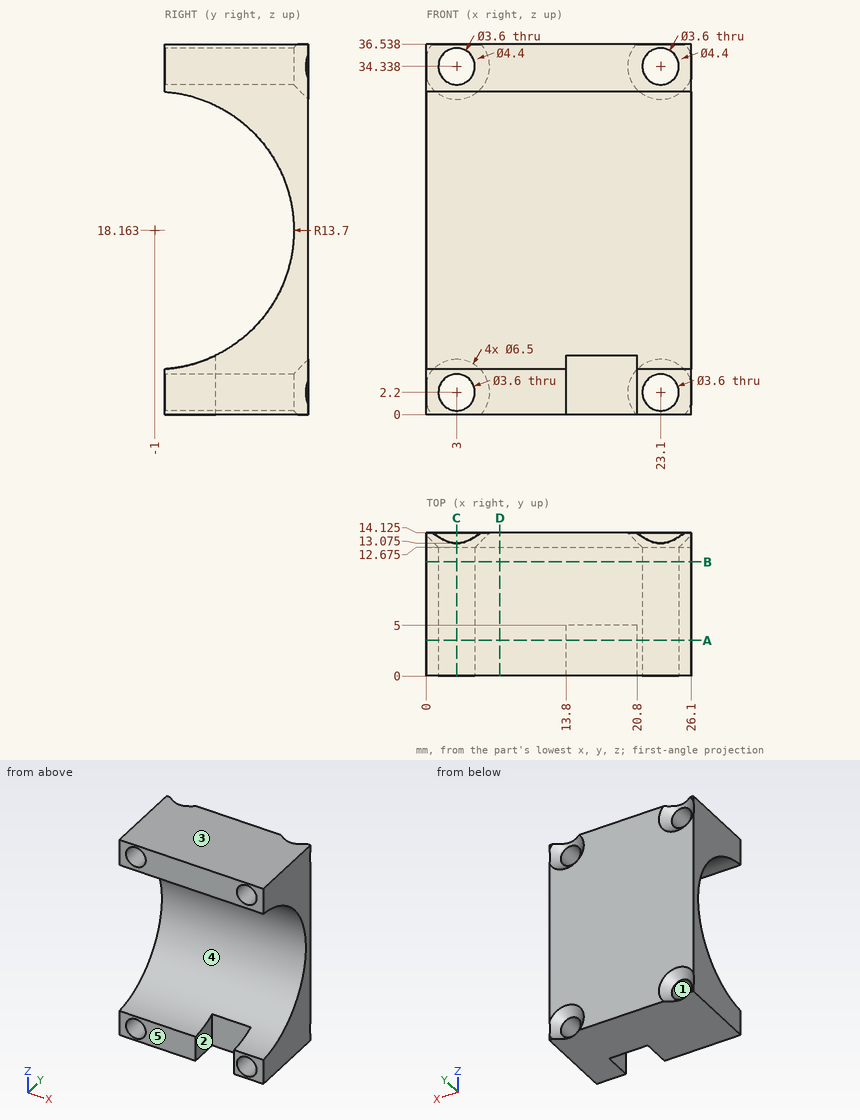
Source: three-view drawing plus pictorial views. Frame: mm from the lowest corner of the part. A direction names the side the tool comes from. Give positions to 0.01 mm unless a question says otherwise; leave off trailing zeros. Order: outer loops, then holes, each group sorted by start corner. A loop starts at its lowest first (then second) coordinate and runs counter-clockwise, first axis right, second up. Notation, with made-up numbers: (88, 18.5) -> (115, 18.5) arc R3 ccw to (115, 22.5) -> close; hole circle Ø9 at (75.5, 74.5). An arc over 180 degrees is marked (long way). Use a Markdown table: item, result.
Q1. Material intervals for line 1 (X direction, y = 12, z = 3); line 2 (Z direction, x = 23.1, y = 4.5) (1 decimal); line 3 (Z direction, x = 23.1, y = 10) (1 decimal), sorted ascending. Write a range as [from, to].
A:
| item | result |
|---|---|
| line 1 | [0, 1.39], [4.61, 21.49], [24.71, 26.1] |
| line 2 | [0, 0.4], [4, 5.6], [30.7, 32.5], [36.1, 36.5] |
| line 3 | [0, 0.4], [4, 10], [26.3, 32.5], [36.1, 36.5] |
Q2. Section A-A (y = 3.5). Return the cut outline in (x, z).
A:
| item | result |
|---|---|
| outline | (0, 0) -> (13.8, 0) -> (13.8, 5.22) -> (0, 5.22) -> close; (0, 31.1) -> (26.1, 31.1) -> (26.1, 36.54) -> (0, 36.54) -> close; (20.8, 0) -> (26.1, 0) -> (26.1, 5.22) -> (20.8, 5.22) -> close; hole circle Ø3.6 at (3, 2.2); hole circle Ø3.6 at (3, 34.34); hole circle Ø3.6 at (23.1, 2.2); hole circle Ø3.6 at (23.1, 34.34) |
Q3. Section B-B (y = 11.25). Return the cut outline in (x, z).
A:
| item | result |
|---|---|
| outline | (0, 0) -> (26.1, 0) -> (26.1, 12.03) -> (0, 12.03) -> close; (0, 24.3) -> (26.1, 24.3) -> (26.1, 36.54) -> (0, 36.54) -> close; hole circle Ø3.6 at (3, 2.2); hole circle Ø3.6 at (3, 34.34); hole circle Ø3.6 at (23.1, 2.2); hole circle Ø3.6 at (23.1, 34.34) |
Q4. Access query for the marked faces 1 and 2. Directions: +Z, -Z, +X, -X, +Y, -Y. A direction counts if a zero-diameter tool reaches every point of the face in a straight line with its end or side. Return the directions, or none.
A:
| item | result |
|---|---|
| face 1 | +Y, -Y |
| face 2 | -Z, -Y |
Q5. Section C-C (x = 3). State how many separate pieces and enclosed holes the cut face has, and give its area (3 significant figures).
A:
| item | result |
|---|---|
| separate pieces | 3 |
| enclosed holes | 0 |
| area | 144 mm^2 |
Q6. First-contact query: P1, Ø3, axis at x = 3, z = 2.2, coming from the +Y side; P2, Ø1.5, axis at y = 1.5, z = 1.5, coming from the -X side; P3, Ø1.5, axis at x = 2.5, z = 12, coming from the -Y side; P4, Ø4.5, axis at x = 23.1, z = 2.2, coming from the +Y side (1 decimal). Flat tips, straight axial feed; report the tip coordinate or a pass-through.
A:
| item | result |
|---|---|
| P1 | through |
| P2 | x = 0 |
| P3 | y = 10.83 |
| P4 | y = 13.1 |
Q7. Section D-D (x = 7.25). Return the cut outline in (y, z) (1 decimal), and give its area (3 significant figures).
A:
| item | result |
|---|---|
| outline | (0, 0) -> (14.1, 0) -> (14.1, 36.5) -> (0, 36.5) -> (0, 31.8) arc R13.7 cw to (0, 4.5) -> close |
| area | 249 mm^2 |
Q8. Pull-direction query (Z, two-part tool) for the marked faces 3, 4 and 5; classes: +Z half, -Z half, draft (parallel to the pull), parting line (faces both ways), or undercut.
A:
| item | result |
|---|---|
| face 3 | +Z half |
| face 4 | undercut |
| face 5 | draft |
